Autodesk Inventor part; units mm, degrees
ref_plane "YZ Plane" through (0, 0, 0) normal (1, 0, 0) x (0, 1, 0)
ref_plane "XZ Plane" through (0, 0, 0) normal (0, 1, 0) x (-1, 0, 0)
ref_plane "XY Plane" through (0, 0, 0) normal (0, 0, 1) x (1, 0, 0)
sketch "Sketch1" plane through (0, 0, 0) normal (0, 1, 0) x (-1, 0, 0)
  circle A0 centre (0, 0) radius 31.75
  circle A1 centre (0, 0) radius 25.527
  dimension "d0" = 63.5
  dimension "d1" = 6.223
extrude "Extrusion1" add sketch "Sketch1" along normal blind 6.35
sketch "Sketch2" plane through (0, 6.35, 0) normal (0, 1, 0) x (1, 0, 0)
  circle A0 centre (0, 0) radius 25.527
  circle A1 centre (0, 28.575) radius 1.535
  dimension "d4" = 28.575
hole "Hole1" at (0, 6.35, -28.575) direction (0, -1, 0) diameter 3.3528 depth 25.4 tip angle 118
pattern_circular "Circular Pattern1" count 4 over 360 about axis through (0, 0, 0) along (0, 1, 0) of "Hole1"
sketch "Sketch4" plane through (0, 0, 0) normal (0, -1, 0) x (1, 0, 0)
  circle A0 centre (0, 0) radius 25.527
  circle A1 centre (0, 0) radius 24.765
  dimension "d16" = 0.762
extrude "Extrusion2" add sketch "Sketch4" against normal blind 137.16
sketch "Sketch5" plane through (0, 137.16, 0) normal (0, 1, 0) x (1, 0, 0)
  circle A0 centre (0, 0) radius 24.765
extrude "Extrusion3" add sketch "Sketch5" against normal blind 4.826
sketch "Sketch6" plane through (0, 137.16, 0) normal (0, 1, 0) x (1, 0, 0)
  circle A0 centre (0, 0) radius 25.527
  circle A1 centre (-10.414, 10.922) radius 4.445
  line L0 (0, 0) -> (-12.3032, 0) construction
  circle A2 centre (-10.414, -10.922) radius 4.445
  dimension "d21" = 10.414
  dimension "d22" = 10.922
  dimension "d23" = 8.89
extrude "Extrusion4" add sketch "Sketch6" along normal blind 12.7 contours A1 | A2
properties part number "balun" material "Copper"
Here's how the part is built. I have some questions about the finished solid (model axes, mm). A direction names the side the tool comes from. Round coordinates to 2 decimals unless told otherwise and drop trailing zeros. Order: outer loops, then holes, each group sorted by start corner. A loop starts at its lowest first (then second) coordinate and runs counter-clockwise, first axis right, second up. Notation, with made-up numbers: (45, -37.5) -> (81, -37.5) arc R27 ccw to (81, -21.5) -> close; hole circle Ø6 at (85.25, 53). An arc over 180 degrees is marked (long way). Use CSV: the item, a comma, the result in double quotes.
1. I want a section at A-A on z = 0. List the corners of the cut face in (x, y) for me (3 decimals), and give its area (3 significant figures).
Recorded:
outline,"(-31.75, 0) -> (-30.251, 0) -> (-30.251, 6.35) -> (-31.75, 6.35) -> close; (-26.899, 0) -> (-24.765, 0) -> (-24.765, 132.334) -> (24.765, 132.334) -> (24.765, 0) -> (26.899, 0) -> (26.899, 6.35) -> (25.527, 6.35) -> (25.527, 137.16) -> (-25.527, 137.16) -> (-25.527, 6.35) -> (-26.899, 6.35) -> close; (30.251, 0) -> (31.75, 0) -> (31.75, 6.35) -> (30.251, 6.35) -> close"
area,"485 mm2"
2. I want a section at B-B on x = 0. List the corners of the cut face in (y, z) for me (3 decimals).
Recorded:
outline,"(0, -31.75) -> (6.35, -31.75) -> (6.35, -30.251) -> (0, -30.251) -> close; (0, -26.899) -> (6.35, -26.899) -> (6.35, -25.527) -> (137.16, -25.527) -> (137.16, 25.527) -> (6.35, 25.527) -> (6.35, 26.899) -> (0, 26.899) -> (0, 24.765) -> (132.334, 24.765) -> (132.334, -24.765) -> (0, -24.765) -> close; (0, 30.251) -> (6.35, 30.251) -> (6.35, 31.75) -> (0, 31.75) -> close"
3. I want a section at D-D on x = 11. List the corners of the cut face in (y, z) for me.
Recorded:
outline,"(0, -29.78) -> (6.35, -29.78) -> (6.35, -23.04) -> (137.16, -23.04) -> (137.16, 23.04) -> (6.35, 23.04) -> (6.35, 29.78) -> (0, 29.78) -> (0, 22.19) -> (132.33, 22.19) -> (132.33, -22.19) -> (0, -22.19) -> close"
4. Which directions (+Z, -Z, +X, -X, +Y, -Y) give clear straight access to the entire face, cutting with the end or side of a thin tool? Please do faces 1 (the face through (0, 6.35, -26)), 2 (the face through (-0.07, 3.13, -30.25)), 3 (the face through (0, 132.334, 0)).
Recorded:
face 1,"+Y"
face 2,"+Y, -Y"
face 3,"-Y"
5. I want a section at C-C on y = 102. List the corners of the cut face in (x, z) for me (3 decimals), and give its area (3 significant figures).
Recorded:
outline,"circle Ø51.054 at (0, 0); hole circle Ø49.53 at (0, 0)"
area,"120 mm2"
6. Thinking about a two-plate mould opening in Z: for faces 4 (the face through (-10.993, 143.421, -6.515)), 5 (the face through (24.348, 70.839, 7.668)), 6 (the face through (23.62, 65.24, 7.44)), 7 (the face through (-10, 149.86, 11)), which applies, pulls with the +Z half, pulls with the -Z half, needs draft (parallel to the pull), parting line crosses it, or undercut?
Recorded:
face 4,"undercut"
face 5,"parting line crosses it"
face 6,"undercut"
face 7,"needs draft"
7. I'm going to push flat-ended pins straight in: P1, Ø5.5, axis at x = 0, z = 28.575, coming from the +Y side; P2, Ø4, axis at x = 0, z = -28.575, coming from the -Y side; P3, Ø12, axis at x = -22, y = 58.5, coming from the -Z side; P4, Ø1, axis at x = -23, y = 127, coming from the +Z side. Where does each tip first touch, or does it pass through?
Recorded:
P1,"stops at y = 6.35"
P2,"stops at y = 0"
P3,"stops at z = -19.89"
P4,"stops at z = 12.06"
8. I need wall thicknesses on line 1 along X through (y, z) = (97, 0) (3 decimals); line 2 along Y through (x, z) = (20.5, 21); line 3 along Z through (x, y) = (9, 29). Which ranges of each line are inside material? Lowest first, please.
Recorded:
line 1,"x = -25.527 to -24.765, 24.765 to 25.527"
line 2,"y = 0 to 6.35"
line 3,"z = -23.89 to -23.07, 23.07 to 23.89"
